Design review of the part built by this model. Coordinates are the model's own, in mm. A direction names the side the tool comes from. Round coordinates to 2 decimals unless told otherwise and drop trailing zeros. Loops run counter-clockwise (first coordinate to the right, second up) from the corner with the lowest first, then second, coordinate; pieces in that order, holes last. Notation, with made-up numbers: (40, 24) -> (62, 24) arc R26 ccw to (62, 38) -> close; hole circle Ø10 at (-28, 68.25). An arc over 180 degrees is marked (long way). Answer as CSV lines item,"result". Start each with the question number.
(1) Draft analysis for pull direction Y (two halves, no side actions). For faces 4 (the face through (49, 81, 3)), 5 (the face through (92, 65.1, 2)), 6 (the face through (96.28, 2.59, -1.3)), state which applies: +Y half, -Y half, draft (parallel to the pull), parting line (faces both ways), or undercut.
(2) Take a section at D-D, the plane y = 68.5. Write out the cut boundary in (x, z), and give its area (3 significant figures).
(3) To check wall thickness, follow line 1 (Y direction, x = 3.2, z = -1.2); line 2 (X direction, y = 79.4, z = -1.4); line 3 (Y direction, x = 80.75, z = -1). State the ranges of each line that lie inside material, in increasing order. Write a range as from..to.
(4) For P1, Ø1, axis at x = 87.5, y = 40, coming from the +Z side; P2, Ø2.5, axis at x = 92, z = 2, coming from the +Y side; P3, Ø1.3, axis at x = 86, z = 1, coming from the -Y side, all flat-tipped, find the tip position at first contact; note any pin that passes through.
(5) Take a section at A-A, the plane y = 3.2. Write out the cut boundary in (x, z), and give its area (3 significant figures).
(6) Take a section at C-C, the plane x = 13. Write out the cut boundary in (y, z), and give its area (3 significant figures).
(7) Machinability: for faces 1 (the face through (5.05, 50, 2)), 2 (the face through (65, 81, 2)), 3 (the face through (6, 50, 3)), which of the approach directions +Z, -Z, +X, -X, +Y, -Y give a long, thin tool a straight path to every point of the face, cutting with its end or side? Answer none if there is none.
(8) Take a section at B-B, the plane x = 3.2. Write out the cut boundary in (y, z).
from build123d import *

# Parameters (mm, degrees)
F0_W     = 98
F0_H     = 82.6
F0_R     = 1.6
F2_DEPTH = 1.6
F1_R     = 5
F3_DEPTH = 1.601
F5_START = -36.1
F5_DEPTH = 29
F7_START = 33
F7_DEPTH = 32
F1_W     = 10
F1_H     = 1.2
F8_DEPTH = 1.2
F9_SIZE  = 1


with BuildPart() as f2:
    # F0 (on Top) → F2 (new body)
    with BuildSketch(Plane.XY):
        with Locations((49, 41.3)):
            Rectangle(F0_W, F0_H)
        with Locations((3.2, 3.2)):
            Circle(F0_R, mode=Mode.SUBTRACT)
        with Locations((94.8, 3.2)):
            Circle(F0_R, mode=Mode.SUBTRACT)
        with Locations((3.2, 79.4)):
            Circle(F0_R, mode=Mode.SUBTRACT)
        with Locations((94.8, 79.4)):
            Circle(F0_R, mode=Mode.SUBTRACT)
    extrude(amount=-F2_DEPTH)

    # F1 (on face) → F3 (cut, through all)
    with BuildSketch(Plane.XY):
        with Locations((80.75, 58.1)):
            Circle(F1_R)
    extrude(amount=-F3_DEPTH, mode=Mode.SUBTRACT)

    # F4 (on Front) → F5 (join)
    with BuildSketch(Plane.XZ.offset(F5_START)):
        with BuildLine():
            add(Edge.make_bspline(
                [(6.25, 0.9831411553), (6.1998556443, 0.4976120788), (6.25, 0.0696883488), (6.25, 0)],
                knots=[1.5113210061, 1.5113210061, 1.5113210061, 1.5113210061, 2.6925824036, 2.6925824036, 2.6925824036, 2.6925824036], degree=3))
            Line((6.25, 0), (6.25, 0.9831411553))
        make_face()
        with BuildLine():
            Line((5.05, 0), (6.25, 0))
            add(Edge.make_bspline(
                [(6.25, 0.9831411553), (6.1998556443, 0.4976120788), (6.25, 0.0696883488), (6.25, 0)],
                knots=[1.5113210061, 1.5113210061, 1.5113210061, 1.5113210061, 2.6925824036, 2.6925824036, 2.6925824036, 2.6925824036], degree=3))
            Line((6.25, 0.9831411553), (6.25, 3))
            Line((6.25, 3), (5.05, 3))
            Line((5.05, 3), (5.05, 0))
        make_face()
        with BuildLine():
            Line((6.25, 3), (6.25, 0.9831411553))
            add(Edge.make_bspline(
                [(7.25, 2.5), (6.5424729796, 2.3198194624), (6.3141553328, 1.6043332928), (6.25, 0.9831411553)],
                knots=[0, 0, 0, 0, 1.5113210061, 1.5113210061, 1.5113210061, 1.5113210061], degree=3))
            Line((7.25, 2.5), (7.25, 3))
            Line((7.25, 3), (6.25, 3))
        make_face()
        with BuildLine():
            Line((92.05, 0.9831411553), (92.05, 3))
            Line((92.05, 3), (91.05, 3))
            Line((91.05, 3), (91.05, 2.5))
            add(Edge.make_bspline(
                [(91.05, 2.5), (91.7575270204, 2.3198194624), (91.9858446672, 1.6043332928), (92.05, 0.9831411553)],
                knots=[0, 0, 0, 0, 1.5113210061, 1.5113210061, 1.5113210061, 1.5113210061], degree=3))
        make_face()
        with BuildLine():
            Line((93.25, 3), (92.05, 3))
            Line((92.05, 3), (92.05, 0.9831411553))
            add(Edge.make_bspline(
                [(92.05, 0.9831411553), (92.1001443557, 0.4976120788), (92.05, 0.0696883488), (92.05, 0)],
                knots=[1.5113210061, 1.5113210061, 1.5113210061, 1.5113210061, 2.6925824036, 2.6925824036, 2.6925824036, 2.6925824036], degree=3))
            Line((92.05, 0), (93.25, 0))
            Line((93.25, 0), (93.25, 3))
        make_face()
        with BuildLine():
            add(Edge.make_bspline(
                [(92.05, 0.9831411553), (92.1001443557, 0.4976120788), (92.05, 0.0696883488), (92.05, 0)],
                knots=[1.5113210061, 1.5113210061, 1.5113210061, 1.5113210061, 2.6925824036, 2.6925824036, 2.6925824036, 2.6925824036], degree=3))
            Line((92.05, 0.9831411553), (92.05, 0))
        make_face()
    extrude(amount=-F5_DEPTH)

    # F6 (on Right) → F7 (join)
    with BuildSketch(Plane.YZ.offset(F7_START)):
        with BuildLine():
            add(Edge.make_bspline(
                [(80.6190222502, 1.5), (80.7199138112, 0.9911874772), (80.6190222502, 0.2993458475), (80.6190222502, 0)],
                knots=[0.4926390921, 0.4926390921, 0.4926390921, 0.4926390921, 1, 1, 1, 1], degree=3))
            Line((80.6190222502, 0), (81.8190222502, 0))
            Line((81.8190222502, 0), (81.8190222502, 3))
            Line((81.8190222502, 3), (80.6190222502, 3))
            Line((80.6190222502, 3), (80.6190222502, 1.5))
        make_face()
        with BuildLine():
            Line((80.6190222502, 1.5), (80.6190222502, 0))
            add(Edge.make_bspline(
                [(80.6190222502, 1.5), (80.7199138112, 0.9911874772), (80.6190222502, 0.2993458475), (80.6190222502, 0)],
                knots=[0.4926390921, 0.4926390921, 0.4926390921, 0.4926390921, 1, 1, 1, 1], degree=3))
        make_face()
        with BuildLine():
            add(Edge.make_bspline(
                [(79.6190222502, 2.5), (80.2328512073, 2.3155356757), (80.5210582047, 1.9940485863), (80.6190222502, 1.5)],
                knots=[0, 0, 0, 0, 0.4926390921, 0.4926390921, 0.4926390921, 0.4926390921], degree=3))
            Line((80.6190222502, 1.5), (80.6190222502, 3))
            Line((80.6190222502, 3), (79.6190222502, 3))
            Line((79.6190222502, 3), (79.6190222502, 2.5))
        make_face()
    extrude(amount=F7_DEPTH)

    # F1 (on face) → F8 (join)
    with BuildSketch(Plane.XY):
        with Locations((11.25, 21)):
            Rectangle(F1_W, F1_H)
        with Locations((86.75, 21)):
            Rectangle(F1_W, F1_H)
    extrude(amount=F8_DEPTH)

    # F9
    f9_edges = [f2.edges().sort_by_distance(p)[0] for p in [
        (1.6, 79.4, 0),
        (1.6, 3.2, 0),
        (93.2, 3.2, 0),
        (93.2, 79.4, 0),
    ]]
    chamfer(f9_edges, length=F9_SIZE)


solid = f2.part
The answers:
1,face 4,"draft"
1,face 5,"+Y half"
1,face 6,"undercut"
2,outline,"(0, -1.6) -> (98, -1.6) -> (98, 0) -> (0, 0) -> close"
2,area,"157 mm²"
3,line 1,"0..1.6, 4.8..77.8, 81..82.6"
3,line 2,"0..1.6, 4.8..93.2, 96.4..98"
3,line 3,"0..53.1, 63.1..82.6"
4,P1,"z = 0"
4,P2,"y = 65.1"
4,P3,"y = 20.4"
5,outline,"(0, -1.6) -> (1.6, -1.6) -> (1.6, -1) -> (0.6, 0) -> (0, 0) -> close; (4.8, -1.6) -> (93.2, -1.6) -> (93.2, -1) -> (92.2, 0) -> (5.8, 0) -> (4.8, -1) -> close; (96.4, -1.6) -> (98, -1.6) -> (98, 0) -> (97.4, 0) -> (96.4, -1) -> close"
5,area,"145 mm²"
6,outline,"(0, -1.6) -> (82.6, -1.6) -> (82.6, 0) -> (21.6, 0) -> (21.6, 1.2) -> (20.4, 1.2) -> (20.4, 0) -> (0, 0) -> close"
6,area,"134 mm²"
7,face 1,"+Z, -X, +Y, -Y"
7,face 2,"+Z, +X, +Y, -Y"
7,face 3,"+Z, +X, -X, +Y, -Y"
8,outline,"(0, -1.6) -> (1.6, -1.6) -> (1.6, -1) -> (0.6, 0) -> (0, 0) -> close; (4.8, -1.6) -> (77.8, -1.6) -> (77.8, -1) -> (76.8, 0) -> (5.8, 0) -> (4.8, -1) -> close; (81, -1.6) -> (82.6, -1.6) -> (82.6, 0) -> (82, 0) -> (81, -1) -> close"
